```python
from build123d import *

# Parameters (mm, degrees)
SKETCH_1_R               = 2
EXTRUDE_1_DEPTH          = 4
CUT_EXTRUDE_1_DEPTH      = 202.596130915
CUT_EXTRUDE_1_DEPTH_BACK = 202.596130915
CUT_EXTRUDE_2_DEPTH      = 202.596130915
CUT_EXTRUDE_2_DEPTH_BACK = 202.596130915
SKETCH_3_R               = 2.1
SKETCH_4_W               = 8
SKETCH_4_H               = 120
EXTRUDE_2_DEPTH          = 4
CUT_EXTRUDE_4_DEPTH      = 208.231754324
CUT_EXTRUDE_4_DEPTH_BACK = 208.231754324
SKETCH_6_R               = 2
CUT_EXTRUDE_5_DEPTH      = 208.231754324
CUT_EXTRUDE_6_DEPTH      = 221.692093198
CUT_EXTRUDE_6_DEPTH_BACK = 221.692093198
SKETCH_9_R               = 1.5
FILLET_1_R               = 2
FILLET_2_R               = 25
SKETCH_11_R              = 2.1
CUT_EXTRUDE_7_DEPTH      = 10


with BuildPart() as part:
    # 草图1 → 凸台-拉伸1 (new body)
    with BuildSketch(Plane(origin=(0, 0, 0), x_dir=(1, 0, 0), z_dir=(0, 1, 0))):
        Polygon((-90, -145), (90, -145), (90, -65), (140, -65), (140, 55), (90, 55), (90, 135), (-90, 135), (-90, 55), (-140, 55), (-140, -65), (-90, -65), align=None)
        with Locations(Location((-83, -138, 0), (0, 0, 270))):
            Circle(SKETCH_1_R, mode=Mode.SUBTRACT)
        with Locations(Location((-83, 128, 0), (0, 0, 270))):
            Circle(SKETCH_1_R, mode=Mode.SUBTRACT)
        with Locations(Location((83, -138, 0), (0, 0, 90))):
            Circle(SKETCH_1_R, mode=Mode.SUBTRACT)
        with Locations(Location((83, 128, 0), (0, 0, 90))):
            Circle(SKETCH_1_R, mode=Mode.SUBTRACT)
        with Locations(Location((-133, 48, 0), (0, 0, 270))):
            Circle(SKETCH_1_R, mode=Mode.SUBTRACT)
        with Locations(Location((-133, -58, 0), (0, 0, 270))):
            Circle(SKETCH_1_R, mode=Mode.SUBTRACT)
        with Locations(Location((-20, 48, 0), (0, 0, 270))):
            Circle(SKETCH_1_R, mode=Mode.SUBTRACT)
        with Locations(Location((-20, -58, 0), (0, 0, 270))):
            Circle(SKETCH_1_R, mode=Mode.SUBTRACT)
    extrude(amount=EXTRUDE_1_DEPTH)

    # 草图2 → 切除-拉伸1 (cut, two sides: drawn at the far end of the back side and taken through both)
    with BuildSketch(Plane(origin=(0, 4, 0), x_dir=(1, 0, 0), z_dir=(0, 1, 0)).offset(-CUT_EXTRUDE_1_DEPTH_BACK)):
        with BuildLine():
            Line((-74, -117), (-44, -117))
            ThreePointArc((-44, -117), (-42, -119), (-44, -121))
            Line((-44, -121), (-74, -121))
            ThreePointArc((-74, -121), (-76, -119), (-74, -117))
        make_face()
        with BuildLine():
            Line((-74, -87), (-44, -87))
            ThreePointArc((-44, -87), (-42, -89), (-44, -91))
            Line((-44, -91), (-74, -91))
            ThreePointArc((-74, -91), (-76, -89), (-74, -87))
        make_face()
        with BuildLine():
            Line((74, -87), (44, -87))
            ThreePointArc((44, -87), (42, -89), (44, -91))
            Line((44, -91), (74, -91))
            ThreePointArc((74, -91), (76, -89), (74, -87))
        make_face()
        with BuildLine():
            Line((74, -117), (44, -117))
            ThreePointArc((44, -117), (42, -119), (44, -121))
            Line((44, -121), (74, -121))
            ThreePointArc((74, -121), (76, -119), (74, -117))
        make_face()
        with BuildLine():
            Line((74, 107), (44, 107))
            ThreePointArc((44, 107), (42, 109), (44, 111))
            Line((44, 111), (74, 111))
            ThreePointArc((74, 111), (76, 109), (74, 107))
        make_face()
        with BuildLine():
            Line((74, 77), (44, 77))
            ThreePointArc((44, 77), (42, 79), (44, 81))
            Line((44, 81), (74, 81))
            ThreePointArc((74, 81), (76, 79), (74, 77))
        make_face()
        with BuildLine():
            Line((-74, 77), (-44, 77))
            ThreePointArc((-44, 77), (-42, 79), (-44, 81))
            Line((-44, 81), (-74, 81))
            ThreePointArc((-74, 81), (-76, 79), (-74, 77))
        make_face()
        with BuildLine():
            Line((-74, 107), (-44, 107))
            ThreePointArc((-44, 107), (-42, 109), (-44, 111))
            Line((-44, 111), (-74, 111))
            ThreePointArc((-74, 111), (-76, 109), (-74, 107))
        make_face()
    extrude(amount=CUT_EXTRUDE_1_DEPTH + CUT_EXTRUDE_1_DEPTH_BACK, mode=Mode.SUBTRACT)

    # 草图3 → 切除-拉伸2 (cut, two sides: drawn at the far end of the back side and taken through both)
    with BuildSketch(Plane(origin=(0, 4, 0), x_dir=(1, 0, 0), z_dir=(0, 1, 0)).offset(-CUT_EXTRUDE_2_DEPTH_BACK)):
        with Locations(Location((-80, 17.529194913, 0), (0, 0, 270))):
            Circle(SKETCH_3_R)
        with Locations(Location((-80, -9, 0), (0, 0, 270))):
            Circle(SKETCH_3_R)
    extrude(amount=CUT_EXTRUDE_2_DEPTH + CUT_EXTRUDE_2_DEPTH_BACK, mode=Mode.SUBTRACT)

    # 草图4 → 凸台-拉伸2 (add)
    with BuildSketch(Plane(origin=(0, 4, 0), x_dir=(1, 0, 0), z_dir=(0, 1, 0))):
        with Locations((144, -5)):
            Rectangle(SKETCH_4_W, SKETCH_4_H)
    extrude(amount=-EXTRUDE_2_DEPTH)

    # 草图6 → 切除-拉伸4 (cut, two sides: drawn at the far end of the back side and taken through both)
    with BuildSketch(Plane.XZ.offset(-CUT_EXTRUDE_4_DEPTH_BACK)):
        with Locations(Location((141, 58, 0), (0, 0, 270))):
            Circle(SKETCH_6_R)
        with Locations(Location((141, -48, 0), (0, 0, 270))):
            Circle(SKETCH_6_R)
    extrude(amount=CUT_EXTRUDE_4_DEPTH + CUT_EXTRUDE_4_DEPTH_BACK, mode=Mode.SUBTRACT)

    # 草图7 → 切除-拉伸5 (cut, through all)
    with BuildSketch(Plane(origin=(0, 4, 0), x_dir=(1, 0, 0), z_dir=(0, 1, 0))):
        with BuildLine():
            Line((-26, -87), (-26, -132))
            ThreePointArc((-26, -132), (-29, -135), (-32, -132))
            Line((-32, -132), (-32, -87))
            ThreePointArc((-32, -87), (-29, -84), (-26, -87))
        make_face()
        with BuildLine():
            Line((32, -87), (32, -132))
            ThreePointArc((32, -132), (29, -135), (26, -132))
            Line((26, -132), (26, -87))
            ThreePointArc((26, -87), (29, -84), (32, -87))
        make_face()
    extrude(amount=-CUT_EXTRUDE_5_DEPTH, mode=Mode.SUBTRACT)

    # 草图9 → 切除-拉伸6 (cut, two sides: drawn at the far end of the back side and taken through both)
    with BuildSketch(Plane(origin=(0, 76, 0), x_dir=(1, 0, 0), z_dir=(0, 1, 0)).offset(-CUT_EXTRUDE_6_DEPTH_BACK)):
        with Locations(Location((72, -38, 0), (0, 0, 180))):
            Circle(SKETCH_9_R)
        with Locations(Location((-2, -38, 0), (0, 0, 180))):
            Circle(SKETCH_9_R)
        with Locations(Location((72, 36, 0), (0, 0, 180))):
            Circle(SKETCH_9_R)
        with Locations(Location((-2, 36, 0), (0, 0, 180))):
            Circle(SKETCH_9_R)
        with Locations(Location((80, -46, 0), (0, 0, 180))):
            Circle(SKETCH_9_R)
        with Locations(Location((-10, -46, 0), (0, 0, 180))):
            Circle(SKETCH_9_R)
        with Locations(Location((-10, 44, 0), (0, 0, 180))):
            Circle(SKETCH_9_R)
        with Locations(Location((80, 44, 0), (0, 0, 180))):
            Circle(SKETCH_9_R)
    extrude(amount=CUT_EXTRUDE_6_DEPTH + CUT_EXTRUDE_6_DEPTH_BACK, mode=Mode.SUBTRACT)

    # 圆角1
    fillet_1_edges = [part.edges().sort_by_distance(p)[0] for p in [
        (148, 2, -55),
        (148, 2, 65),
        (90, 2, 145),
        (-90, 2, 145),
        (-140, 2, 65),
        (-140, 2, -55),
        (-90, 2, -135),
        (90, 2, -135),
    ]]
    fillet(fillet_1_edges, radius=FILLET_1_R)

    # 圆角2
    fillet_2_edges = [part.edges().sort_by_distance(p)[0] for p in [
        (90, 2, -55),
        (90, 2, 65),
        (-90, 2, 65),
        (-90, 2, -55),
    ]]
    fillet(fillet_2_edges, radius=FILLET_2_R)

    # 草图11 → 切除-拉伸7 (cut)
    with BuildSketch(Plane(origin=(0, 4, 0), x_dir=(1, 0, 0), z_dir=(0, 1, 0))):
        with Locations(Location((-13, -131.714712401, 0), (0, 0, 270))):
            Circle(SKETCH_11_R)
        with Locations(Location((13, -130.851588753, 0), (0, 0, 270))):
            Circle(SKETCH_11_R)
        with Locations(Location((13, -93.714712401, 0), (0, 0, 270))):
            Circle(SKETCH_11_R)
        with Locations(Location((-13, -93.714712401, 0), (0, 0, 270))):
            Circle(SKETCH_11_R)
    extrude(amount=-CUT_EXTRUDE_7_DEPTH, mode=Mode.SUBTRACT)


solid = part.part
```
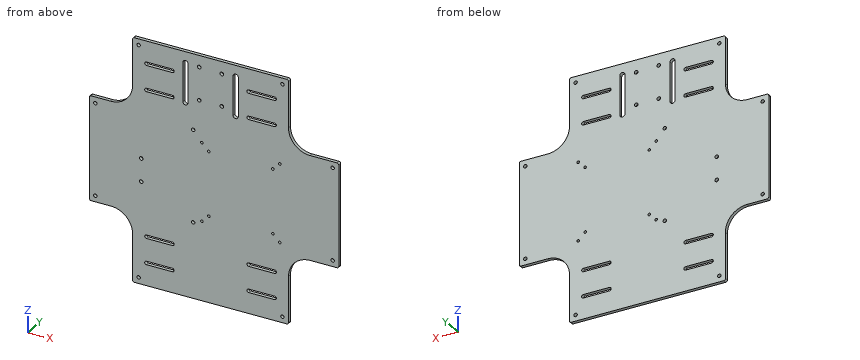
Design review of the part built by this model. Coordinates are the model's own, in mm. Coordinates: 2 decimals unless noted, no trailing zeros. Order: outer loops, then holes, each group sorted by start corner. A loop starts at its lowest first (then second) coordinate and runs counter-clockwise, first axis right, second up. Notation, with made-up numbers: (12.5, 30.5) - (34.5, 30.5) arc R18 cw to (34.5, 47.5) - close; hole circle Ø6 at (4, 78). An arc over 180 degrees is marked (long way). Answer in a Markdown table with one row per item.
(1) Consider section B-B on y = 0.8. Give the number of separate pieces and of enclosed holes in the cut face, plus the area to 3 significant figures.
Checked values:
| item | result |
|---|---|
| separate pieces | 1 |
| enclosed holes | 34 |
| area | 62,000 mm^2 |
(2) Wall thickness on line 1 along Z through (x, y) = (63, 1.7); line 2 along Z through (x, y) = (83, 2.85); line 3 along X through (y, z) = (0.9, 122): over which ranges is each line inside the solid? List them lowest first. Write a range as from..to.
Checked values:
| item | result |
|---|---|
| line 1 | -135..-111, -107..-81, -77..87, 91..117, 121..145 |
| line 2 | -135..-130, -126..136, 140..145 |
| line 3 | -90..-32, -26..26, 32..90 |
(3) Clearance check with flat-ended pins moving along their axes: pin 1 (2 mm diameter, centred on y = 1.5, z = 104, fed in from -X); pin 2 (2.5 mm diameter, centred on x = 72, z = 38, fed in from +Y); pin 3 (2 mm diameter, centred on y = 3.5, z = -86, fed in from +X); pin 4 (2 mm diameter, centred on x = 135, y = 2, fed in from +Z). State where each tip first meets the part, or that it passes through.
Checked values:
| item | result |
|---|---|
| pin 1 | x = -90 |
| pin 2 | through |
| pin 3 | x = 90 |
| pin 4 | z = 65 |
(4) Consider section C-C on z = 80.5. State the section outline as (x, y) points.
Checked values:
| item | result |
|---|---|
| outline | (-91.88, 0) - (91.88, 0) - (91.88, 4) - (-91.88, 4) - close |
(5) Consider section A-A on x = -95. State the section outline as (y, z) points, plus the area to 3 significant figures.
Checked values:
| item | result |
|---|---|
| outline | (0, -65) - (4, -65) - (4, 75) - (0, 75) - close |
| area | 560 mm^2 |
